Input: part model. Units: mm. Frame: model coordinates. Face numbers are marked on the shaded views. A direction names the side the tool comes from. Give positions to 0.01 mm unless a question says otherwise; leave off trailing zeros. Loops run counter-clockwise (first coordinate to the right, second up) from the corner with the lowest first, then second, coordinate; pieces in that order, holes last. Notation, with made-up numbers: M 21.25,19 L 46.25,19 A4 cw 46.25,25 Z; hole C 10,87.25 d10. An arc over 180 degrees is marked long. Return JSON: item names as keys, results as strings. Group by question number.
```python
from build123d import *

# Parameters (mm, degrees)
F0_W     = 40
F0_H     = 5
F1_DEPTH = 10
F2_R     = 2.05
F3_DEPTH = 25
F4_R     = 2.05
F5_DEPTH = 25
F6_R     = 4.99999
F7_W     = 20
F7_H     = 6
F8_DEPTH = 25


# Not quite as in the source:
# - a fillet or chamfer is up to 0.001 mm smaller than in the source, because OpenCascade refuses the exact size


with BuildPart() as f1:
    # F0 (on Top) → F1 (new body)
    with BuildSketch(Plane.XY):
        with Locations((20, 2.5)):
            Rectangle(F0_W, F0_H)
    extrude(amount=F1_DEPTH)

    # F2 (on face) → F3 (cut)
    with BuildSketch(Plane.XZ):
        with Locations((5, 5)):
            Circle(F2_R)
    extrude(amount=-F3_DEPTH, mode=Mode.SUBTRACT)

    # F4 (on face) → F5 (cut)
    with BuildSketch(Plane.XZ):
        with Locations((35, 5)):
            Circle(F4_R)
    extrude(amount=-F5_DEPTH, mode=Mode.SUBTRACT)

    # F6 (radius 5 in the source; OpenCascade refuses exactly that, so slightly less here)
    f6_edges = [f1.edges().sort_by_distance(p)[0] for p in [
        (0, 2.5, 10),
        (0, 2.5, 0),
        (40, 2.5, 10),
        (40, 2.5, 0),
    ]]
    fillet(f6_edges, radius=F6_R)

    # F7 (on face) → F8 (cut)
    with BuildSketch(Plane(origin=(0, 5, 0), x_dir=(-1, 0, 0), z_dir=(0, 1, 0))):
        with Locations((-20, 5)):
            Rectangle(F7_W, F7_H)
    extrude(amount=-F8_DEPTH, mode=Mode.SUBTRACT)


solid = f1.part
```
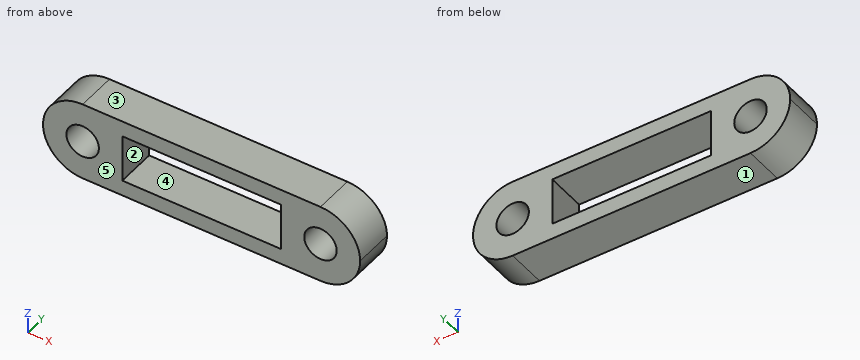
Item 1: Section B-B, the plane x = 21. Return loops of the section in (y, z).
Item 2: Reachability of the marked faces 1 and 2 from +Z, -Z, +X, -X, +Y, -Y: full face, straight path, thin tool, end or side. Return the list, or none.
Item 3: Section C-C, the plane x = 4.5. Return loops of the section in (y, z), then the cut area to 3 significant figures.
Item 4: Section D-D, the plane z = 8.5. Return loops of the section in (x, y).
Item 5: First-contact query: pin 1 Ø2 at (y, z) = (1.5, 8.5) entering from +X; pin 2 Ø5.5 at (x, z) = (5, 5) entering from +Y. Flat tips, straight axial feed; report the tip coordinate or a pass-through.
Item 6: Material intervals for line 1 (Z direction, x = 10.5, y = 1.7); line 2 (Z direction, x = 35, y = 3); line 3 (X direction, y = 3.95, z = 4.5), sorted ascending. Write a range as from..to.
Item 7: Section A-A, the plane y = 1.9. Give the number of separate pieces and of enclosed holes in the cut face, then the cut area to 3 significant figures.
Item 8: Pull-direction query (Z, two-part tool) for the marked faces 3, 4 and 5; classes: pulls with the +Z half, pulls with the -Z half, needs draft (parallel to the pull), parting line crosses it, or undercut.
Answer below:
{
 "1": {"outline": "M 0,0 L 5,0 L 5,2 L 0,2 Z; M 0,8 L 5,8 L 5,10 L 0,10 Z"},
 "2": {"face 1": "-Z, +X, -X, +Y, -Y", "face 2": "+Y, -Y"},
 "3": {"outline": "M 0,0.03 L 5,0.03 L 5,3.01 L 0,3.01 Z; M 0,6.99 L 5,6.99 L 5,9.97 L 0,9.97 Z", "area": "29.9 mm^2"},
 "4": {"outline": "M 1.43,0 L 38.57,0 L 38.57,5 L 1.43,5 Z"},
 "5": {"pin 1": "x = 39.33", "pin 2": "y = 5"},
 "6": {"line 1": "0..2, 8..10", "line 2": "0..2.95, 7.05..10", "line 3": "0.03..3.01, 6.99..10, 30..33.01, 36.99..39.97"},
 "7": {"separate pieces": "1", "enclosed holes": "3", "area": "232 mm^2"},
 "8": {"face 3": "pulls with the +Z half", "face 4": "undercut", "face 5": "needs draft"}
}
